Source: CAD feature listing. Evaluate the final solid. Frame: model axes, mm. A direction names the side the tool comes from. Coordinates: 2 decimals unless noted, no trailing zeros. Order: outer loops, then holes, each group sorted by start corner. A loop starts at its lowest first (then second) coordinate and runs counter-clockwise, first axis right, second up.
Item 1: Section D-D on x = 552. Return the cut outline in (y, z), then the cut area to 3 significant figures.
Item 2: Ray query, line 1 (Z direction, x = -728, y = 113.5); line 2 (X direction, y = 426, z = -126.5); line 3 (Z direction, x = -464, y = 258). Return the intervals inside material, ascending.
Item 3: Section C-C on y = 390.5. Return the cut outline in (x, z), then the cut area to 3 significant figures.
Item 4: Contact query for flat-ended pins moving along their axis: P1, Ø1, axis at x = -652.5, z = 36.5, coming from the +Y side; P2, Ø1.5, axis at y = 89, z = -103.5, coming from the -X side; P3, Ø12.5, axis at x = 856.5, z = -17.5, coming from the +Y side. Output: stop coordinate, or through.
Item 5: Reachability of faces 4 (the cylindrical face through (-257.307, 304.584, 431.089)), 5 (the flat face through (711.2, 337, 5)), 6 (the flat face through (749, 330.2, -2)) from +Z, -Z, +X, -X, +Y, -Y: full face, straight path, thin tool, end or side. Return the list, or none.
Item 6: Mould query, pull axis Y, two halves, no side actions, for faces 1 (the flat face through (863.6, 213, 6)), 2 (the cylindrical face through (-257.307, 304.584, -432.511)), 3 (the cylindrical face through (623.25, 300.82, -432.51)). Classes: released by +Y, released by -Y, zero draft, split by the parting line, or undercut.
Item 7: Section A-A on x = -76.2. Return the cut outline in (y, z), then the cut area to 3 significant figures.
Item 8: Section B-B on z = -38. Return the cut outline in (x, y).
from build123d import *

# Parameters (mm, degrees)
SKETCH1_W               = 1727.2
SKETCH1_H               = 965.2
SKETCH1_W_2             = 1422.4
SKETCH1_H_2             = 762
BOSS_EXTRUDE1_DEPTH     = 457.2
SKETCH2_W               = 1422.4
SKETCH2_H               = 762
BOSS_EXTRUDE2_DEPTH     = 152.4
CUT_EXTRUDE1_DEPTH      = 1374.480192795
CUT_EXTRUDE1_DEPTH_BACK = 1374.480192795
SKETCH4_R               = 25.4
SKETCH7_W               = 304.8
SKETCH7_H               = 127
CUT_EXTRUDE2_DEPTH      = 127
SKETCH8_W               = 76.2
SKETCH8_H               = 304.8
CUT_EXTRUDE3_DEPTH      = 304.8
SKETCH9_W               = 25.4
SKETCH9_H               = 304.8
BOSS_EXTRUDE3_DEPTH     = 25.4
SKETCH11_W              = 304.8
SKETCH11_H              = 127
CUT_EXTRUDE5_DEPTH      = 127
SKETCH13_W              = 25.4
SKETCH13_H              = 304.8
BOSS_EXTRUDE4_DEPTH     = 25.4
SKETCH14_W              = 76.2
SKETCH14_H              = 304.8
CUT_EXTRUDE7_DEPTH      = 279.4
FILLET1_R               = 25.4
FILLET2_R               = 25.4


with BuildPart() as part:
    # Sketch1 → Boss-Extrude1 (new body)
    with BuildSketch(Plane(origin=(0, 0, 0), x_dir=(1, 0, 0), z_dir=(0, 1, 0))):
        Rectangle(SKETCH1_W, SKETCH1_H)
        Rectangle(SKETCH1_W_2, SKETCH1_H_2, mode=Mode.SUBTRACT)
    extrude(amount=BOSS_EXTRUDE1_DEPTH)

    # Sketch2 → Boss-Extrude2 (add)
    with BuildSketch(Plane(origin=(0, 0, 0), x_dir=(1, 0, 0), z_dir=(0, 1, 0))):
        Rectangle(SKETCH2_W, SKETCH2_H)
    extrude(amount=BOSS_EXTRUDE2_DEPTH)

    # Sketch4 → Cut-Extrude1 (cut, two sides: drawn at the far end of the back side and taken through both)
    with BuildSketch(Plane.XY.offset(482.6).offset(-CUT_EXTRUDE1_DEPTH_BACK)):
        with Locations((-609.6, 279.4)):
            Circle(SKETCH4_R)
        with Locations((-431.8, 279.4)):
            Circle(SKETCH4_R)
        with Locations((-254, 279.4)):
            Circle(SKETCH4_R)
        with Locations((-76.2, 279.4)):
            Circle(SKETCH4_R)
        with Locations((76.2, 279.4)):
            Circle(SKETCH4_R)
        with Locations((254, 279.4)):
            Circle(SKETCH4_R)
        with Locations((431.8, 279.4)):
            Circle(SKETCH4_R)
        with Locations((609.6, 279.4)):
            Circle(SKETCH4_R)
    extrude(amount=CUT_EXTRUDE1_DEPTH + CUT_EXTRUDE1_DEPTH_BACK, mode=Mode.SUBTRACT)

    # Sketch7 → Cut-Extrude2 (cut)
    with BuildSketch(Plane(origin=(863.6, 0, 0), x_dir=(0, 0, -1), z_dir=(1, 0, 0))):
        with Locations((0, 88.9)):
            Rectangle(SKETCH7_W, SKETCH7_H)
    extrude(amount=-CUT_EXTRUDE2_DEPTH, mode=Mode.SUBTRACT)

    # Sketch8 → Cut-Extrude3 (cut)
    with BuildSketch(Plane(origin=(0, 25.4, 0), x_dir=(1, 0, 0), z_dir=(0, 1, 0))):
        with Locations((749.3, 0)):
            Rectangle(SKETCH8_W, SKETCH8_H)
    extrude(amount=CUT_EXTRUDE3_DEPTH, mode=Mode.SUBTRACT)

    # Sketch9 → Boss-Extrude3 (add)
    with BuildSketch(Plane(origin=(0, 25.4, 0), x_dir=(1, 0, 0), z_dir=(0, 1, 0))):
        with Locations((850.9, 0)):
            Rectangle(SKETCH9_W, SKETCH9_H)
    extrude(amount=BOSS_EXTRUDE3_DEPTH)

    # Sketch11 → Cut-Extrude5 (cut)
    with BuildSketch(Plane.ZY.offset(863.6)):
        with Locations((0, 88.9)):
            Rectangle(SKETCH11_W, SKETCH11_H)
    extrude(amount=-CUT_EXTRUDE5_DEPTH, mode=Mode.SUBTRACT)

    # Sketch13 → Boss-Extrude4 (add)
    with BuildSketch(Plane(origin=(0, 25.4, 0), x_dir=(1, 0, 0), z_dir=(0, 1, 0))):
        with Locations((-850.9, 0)):
            Rectangle(SKETCH13_W, SKETCH13_H)
    extrude(amount=BOSS_EXTRUDE4_DEPTH)

    # Sketch14 → Cut-Extrude7 (cut)
    with BuildSketch(Plane(origin=(0, 25.4, 0), x_dir=(1, 0, 0), z_dir=(0, 1, 0))):
        with Locations((-749.3, 0)):
            Rectangle(SKETCH14_W, SKETCH14_H)
    extrude(amount=CUT_EXTRUDE7_DEPTH, mode=Mode.SUBTRACT)

    # Fillet1
    fillet1_edges = [part.edges().sort_by_distance(p)[0] for p in [
        (863.6, 457.2, 0),
        (0, 457.2, -482.6),
        (-863.6, 457.2, 0),
        (0, 457.2, 482.6),
    ]]
    fillet(fillet1_edges, radius=FILLET1_R)

    # Fillet2
    # the kernel refuses this fillet: 25.4 mm, written as the material it takes off along each edge
    with BuildSketch(Plane(origin=(-838.2, 431.8, 457.2), x_dir=(0, 0, 1), z_dir=(-1, 0, 0))) as fillet2_piece_1_section:
        Polygon((0, 0), (FILLET2_R * 1.02, 0), (FILLET2_R * 1.02, FILLET2_R * 1.02), (0, FILLET2_R * 1.02), align=None)
    fillet2_piece_1 = extrude(amount=FILLET2_R * 1.02, mode=Mode.PRIVATE)
    fillet2_piece_1 = fillet2_piece_1 - Plane(origin=(-838.2, 431.8, 457.2), x_dir=(0, -0.7071067811865475, -0.7071067811865475), z_dir=(-1, 0, 0)) * Sphere(FILLET2_R, mode=Mode.PRIVATE)
    add(fillet2_piece_1, mode=Mode.SUBTRACT)
    with BuildSketch(Plane(origin=(-838.2, 431.8, -457.2), x_dir=(-1, 0, 0), z_dir=(0, 0, -1))) as fillet2_piece_2_section:
        Polygon((0, 0), (FILLET2_R * 1.02, 0), (FILLET2_R * 1.02, FILLET2_R * 1.02), (0, FILLET2_R * 1.02), align=None)
    fillet2_piece_2 = extrude(amount=FILLET2_R * 1.02, mode=Mode.PRIVATE)
    fillet2_piece_2 = fillet2_piece_2 - Plane(origin=(-838.2, 431.8, -457.2), x_dir=(0.7071067811865475, -0.7071067811865475, 0), z_dir=(0, 0, -1)) * Sphere(FILLET2_R, mode=Mode.PRIVATE)
    add(fillet2_piece_2, mode=Mode.SUBTRACT)
    with BuildSketch(Plane(origin=(838.2, 431.8, 457.2), x_dir=(0, 0, 1), z_dir=(1, 0, 0))) as fillet2_piece_3_section:
        Polygon((0, 0), (FILLET2_R * 1.02, 0), (FILLET2_R * 1.02, -FILLET2_R * 1.02), (0, -FILLET2_R * 1.02), align=None)
    fillet2_piece_3 = extrude(amount=FILLET2_R * 1.02, mode=Mode.PRIVATE)
    fillet2_piece_3 = fillet2_piece_3 - Plane(origin=(838.2, 431.8, 457.2), x_dir=(0, -0.7071067811865475, -0.7071067811865475), z_dir=(1, 0, 0)) * Sphere(FILLET2_R, mode=Mode.PRIVATE)
    add(fillet2_piece_3, mode=Mode.SUBTRACT)
    with BuildSketch(Plane(origin=(838.2, 431.8, -457.2), x_dir=(1, 0, 0), z_dir=(0, 0, -1))) as fillet2_piece_4_section:
        Polygon((0, 0), (FILLET2_R * 1.02, 0), (FILLET2_R * 1.02, -FILLET2_R * 1.02), (0, -FILLET2_R * 1.02), align=None)
    fillet2_piece_4 = extrude(amount=FILLET2_R * 1.02, mode=Mode.PRIVATE)
    fillet2_piece_4 = fillet2_piece_4 - Plane(origin=(838.2, 431.8, -457.2), x_dir=(-0.7071067811865475, -0.7071067811865475, 0), z_dir=(0, 0, -1)) * Sphere(FILLET2_R, mode=Mode.PRIVATE)
    add(fillet2_piece_4, mode=Mode.SUBTRACT)
    with BuildSketch(Plane(origin=(863.6, -63.5, -482.6), x_dir=(-1, 0, 0), z_dir=(0, 1, 0)), Plane(origin=(863.6, -63.5, 482.6), x_dir=(0, 0, -1), z_dir=(0, 1, 0))) as fillet2_piece_5:
        with BuildLine():
            CenterArc((FILLET2_R, FILLET2_R), FILLET2_R, 180, 90)
            Line((0, FILLET2_R), (0, 0))
            Line((0, 0), (FILLET2_R, 0))
        make_face()
    extrude(amount=495.3, mode=Mode.SUBTRACT)
    with BuildSketch(Plane(origin=(-863.6, -63.5, -482.6), x_dir=(1, 0, 0), z_dir=(0, 1, 0)), Plane(origin=(-863.6, -63.5, 482.6), x_dir=(0, 0, -1), z_dir=(0, 1, 0))) as fillet2_piece_6:
        with BuildLine():
            CenterArc((FILLET2_R, -FILLET2_R), FILLET2_R, 90, 90)
            Line((0, -FILLET2_R), (0, 0))
            Line((0, 0), (FILLET2_R, 0))
        make_face()
    extrude(amount=495.3, mode=Mode.SUBTRACT)


solid = part.part
Answer list:
1. outline: (0, -482.6) - (431.8, -482.6) arc R25.4 ccw to (457.2, -457.2) - (457.2, -381) - (152.4, -381) - (152.4, 381) - (457.2, 381) - (457.2, 457.2) arc R25.4 ccw to (431.8, 482.6) - (0, 482.6) - close
1. area: 209,000 mm2
2. line 1: z = -482.6 to -152.4, 152.4 to 482.6
2. line 2: x = -863.6 to -711.2, 711.2 to 863.6
2. line 3: z = -482.6 to -381, 381 to 482.6
3. outline: (-863.6, -457.2) arc R25.4 ccw to (-838.2, -482.6) - (838.2, -482.6) arc R25.4 ccw to (863.6, -457.2) - (863.6, 457.2) arc R25.4 ccw to (838.2, 482.6) - (-838.2, 482.6) arc R25.4 ccw to (-863.6, 457.2) - close; hole (-711.2, -381) - (711.2, -381) - (711.2, 381) - (-711.2, 381) - close
3. area: 583,000 mm2
4. P1: stops at y = 152.4
4. P2: stops at x = -711.2
4. P3: stops at y = 454.16
5. face 4: +Z, -Z
5. face 5: +Y
5. face 6: none
6. face 1: zero draft
6. face 2: undercut
6. face 3: undercut
7. outline: (0, -482.6) - (254, -482.6) - (254, -381) - (152.4, -381) - (152.4, 381) - (254, 381) - (254, 482.6) - (0, 482.6) - close; (304.8, -482.6) - (431.8, -482.6) arc R25.4 ccw to (457.2, -457.2) - (457.2, -381) - (304.8, -381) - close; (304.8, 381) - (457.2, 381) - (457.2, 457.2) arc R25.4 ccw to (431.8, 482.6) - (304.8, 482.6) - close
7. area: 198,000 mm2
8. outline: (-863.6, 0) - (863.6, 0) - (863.6, 50.8) - (838.2, 50.8) - (838.2, 25.4) - (711.2, 25.4) - (711.2, 152.4) - (-711.2, 152.4) - (-711.2, 25.4) - (-838.2, 25.4) - (-838.2, 50.8) - (-863.6, 50.8) - close; (-863.6, 152.4) - (-787.4, 152.4) - (-787.4, 304.8) - (-711.2, 304.8) - (-711.2, 457.2) - (-838.2, 457.2) arc R25.4 ccw to (-863.6, 431.8) - close; (711.2, 330.2) - (787.4, 330.2) - (787.4, 152.4) - (863.6, 152.4) - (863.6, 431.8) arc R25.4 ccw to (838.2, 457.2) - (711.2, 457.2) - close
